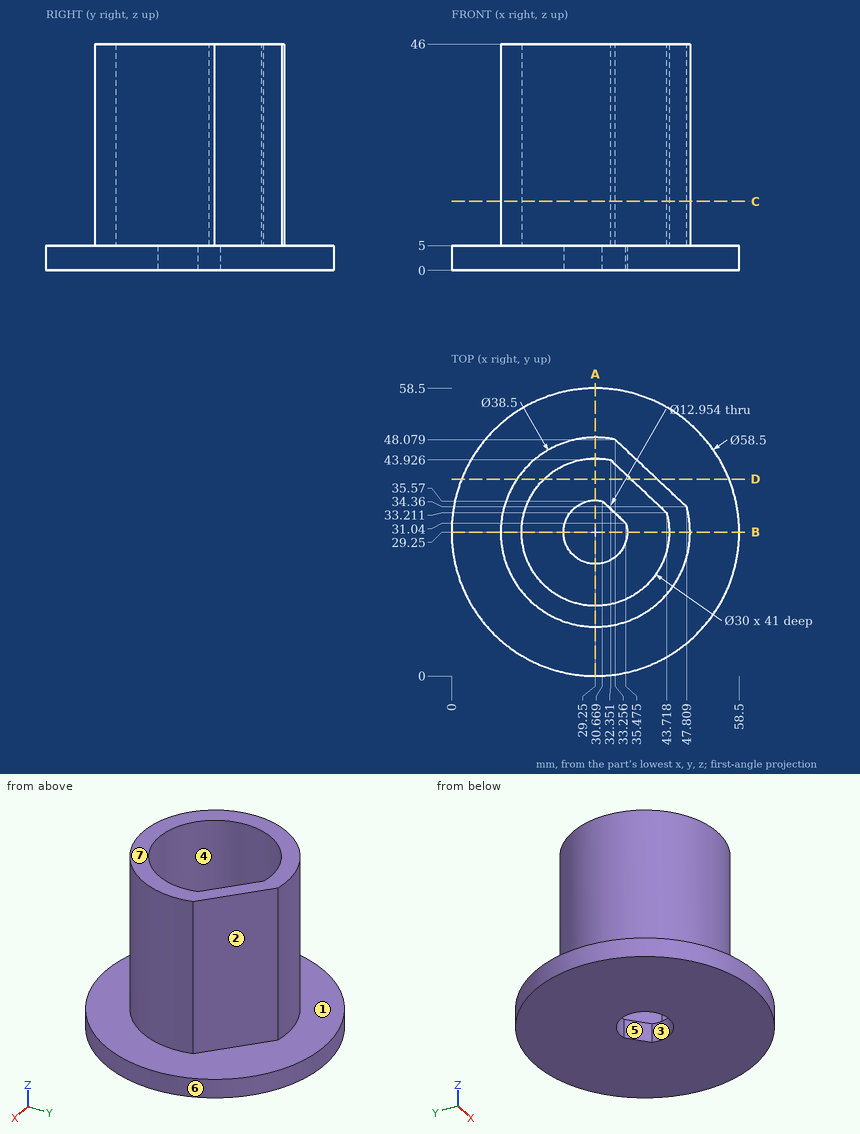
Job drawing, mm, ordinate dimensions from the low corner. One solid piece. A direction names the side the tool comes from. Give positions to 0.01 mm unless a question says otherwise; leave off trailing zeros. Loops run counter-clockwise (first coordinate to the right, second up) from the corner with the lowest first, then second, coordinate; pieces in that order, holes last. Notation, with made-up numbers: (58, 32.5) - (109, 32.5) arc R28 cw to (109, 51.5) - close; hole circle Ø3 at (-2.75, 47). An arc over 180 degrees is marked (long way). Use one line per item in the form item = value.
(1) Cut at A-A (x = 29.25). Give the cut face in (y, z), then the cut area to 3 significant figures.
Determined:
outline = (0, 0) - (22.77, 0) - (22.77, 5) - (14.25, 5) - (14.25, 46) - (10, 46) - (10, 5) - (0, 5) - close; (35.73, 0) - (58.5, 0) - (58.5, 5) - (48.5, 5) - (48.5, 46) - (44.25, 46) - (44.25, 5) - (35.73, 5) - close
area = 576 mm^2
(2) Pull direction Y, two halves, no side cores. Call the marked faces 4, 5, 6 and 7: pulls with the +Y half, pulls with the -Y half, needs draft (parallel to the pull), parting line crosses it, or undercut.
Determined:
face_4 = undercut
face_5 = undercut
face_6 = parting line crosses it
face_7 = needs draft
(3) 3-axis set-ups, long thin cutter, end or side, ignore diameter. For the marked faces 1, 2 and 3: which of +Z, -Z, +X, -X, +Y, -Y reach the whole face in a straight line?
Determined:
face_1 = +Z
face_2 = +Z, +X, +Y
face_3 = +Z, -Z
(4) Drill centre lines: L1, parallel to Y at x = 29.25, z = 2; L2, parallel to Y at x = 29, z = 23; L3, parallel to Z at x = 43.5, y = 25. Where is each one in solid material? Low to high.
Determined:
L1 = 0 to 22.77, 35.73 to 58.5
L2 = 10 to 14.25, 44.25 to 48.5
L3 = 0 to 5
(5) Cut at D-D (y = 40). Give the cut face in (x, z) (1 decimal).
Determined:
outline = (2, 0) - (56.5, 0) - (56.5, 5) - (41.8, 5) - (41.8, 46) - (36.5, 46) - (36.5, 5) - (18.8, 5) - (18.8, 46) - (13.3, 46) - (13.3, 5) - (2, 5) - close
(6) Drop flat-ended pins along their axis: P1, Ø3, axis at y = 26.5, z = 25, coming from the +X side; P2, Ø1.5, axis at y = 51, z = 24, coming from the -X side; P3, Ø2, axis at x = 29.5, z = 34.5, coming from the +Y side; P4, Ø12, axis at y = 8, z = 17, coming from the -X side. Give the stop position or say it passes through.
Determined:
P1 = 48.46
P2 = through
P3 = 48.5
P4 = 17.5
(7) Cut at C-C (z = 14). Give the cut face in (x, y).
Determined:
outline = (33.26, 48.08) arc R19.25 ccw (long way) to (47.81, 34.36) - close; hole (32.35, 43.93) arc R15 ccw (long way) to (43.72, 33.21) - close
